```python
from build123d import *

# Parameters (mm, degrees)
F0_W     = 6
F0_H     = 21
F1_DEPTH = 4
F2_R     = 2
F3_DEPTH = 6
F4_R     = 1
F5_DEPTH = 4


with BuildPart() as f1:
    # F0 (on Top) → F1 (new body)
    with BuildSketch(Plane.XY):
        with Locations((-3, 10.5)):
            Rectangle(F0_W, F0_H)
    extrude(amount=F1_DEPTH)

    # F2 (on face) → F3 (join)
    with BuildSketch(Plane.XY.offset(4)):
        with Locations((-3, 17)):
            Circle(F2_R)
    extrude(amount=F3_DEPTH)

    # F4 (on face) → F5 (cut)
    with BuildSketch(Plane.XZ):
        with Locations((-3, 2)):
            Circle(F4_R)
    extrude(amount=-F5_DEPTH, mode=Mode.SUBTRACT)


solid = f1.part
```
The model under review builds one solid part; all positions refer to its coordinate system, in mm. A direction names the side the tool comes from. Round coordinates to 2 decimals unless told otherwise and drop trailing zeros. Write each loop counter-clockwise with the first axis right and the second up, starting at its lowest first coordinate (ties: lowest second). Pieces come first, ordered by that corner, then holes.
(1) We need section B-B on x = -3. Give the boundary of the cut face in (y, z), and give its area (3 significant figures).
(2) Wall thickness on L1, parallel to Z at x = -3, y = 1.4; L2, parallel to Z at x = -4.05, y = 10.75; L3, parallel to Y at x = -3.3, z = 2: over which ranges is each line inside the solid? List them lowest first.
(3) We need section A-A on y = 3. Give the boundary of the cut face in (x, z).
(4) Insertion check: pin 1 (1.6 mm diameter, centred on x = -3, z = 2, fed in from -Y); pin 2 (3 mm diameter, centred on x = -1, z = 3.5, fed in from -Y); pin 3 (3 mm diameter, centred on x = -4, z = 6, fed in from -Y); pin 4 (3 mm diameter, centred on x = -1.5, y = 10.5, fed in from +Z). Each pin has a flat end and moves straight along its axis. Give the tip position at first contact, or say it passes through.
(5) Mouldability with a two-part tool opening along Z and no side actions: class faces 4 (the flat face through (0, 10, 2)), 5 (the flat face through (-3, 11, 0)), 6 (the cylindrical face through (-3, 2, 1)) as +Z half, -Z half, draft (parallel to the pull), parting line (faces both ways), or undercut.
(6) We need section C-C on z = 2. Give the boundary of the cut face in (x, y).
(7) We need section D-D on y = 17. Give the boundary of the cut face in (x, z).
(8) Machinability: for faces 1 (the flat face through (-6, 10, 2)), 2 (the cylindrical face through (-3, 19, 7)), 3 (the flat face through (-3, 4, 2)), which of the approach directions +Z, -Z, +X, -X, +Y, -Y give a long, thin tool a straight path to every point of the face, cutting with its end or side? Answer none if there is none.
Findings below:
1. outline: (0, 0) - (21, 0) - (21, 4) - (19, 4) - (19, 10) - (15, 10) - (15, 4) - (0, 4) - (0, 3) - (4, 3) - (4, 1) - (0, 1) - close
1. area: 100 mm2
2. L1: z = 0 to 1, 3 to 4
2. L2: z = 0 to 4
2. L3: y = 4 to 21
3. outline: (-6, 0) - (0, 0) - (0, 4) - (-6, 4) - close; hole circle Ø2 at (-3, 2)
4. pin 1: stops at y = 4
4. pin 2: stops at y = 0
4. pin 3: stops at y = 15
4. pin 4: stops at z = 4
5. face 4: draft
5. face 5: -Z half
5. face 6: undercut
6. outline: (-6, 0) - (-4, 0) - (-4, 4) - (-2, 4) - (-2, 0) - (0, 0) - (0, 21) - (-6, 21) - close
7. outline: (-6, 0) - (0, 0) - (0, 4) - (-1, 4) - (-1, 10) - (-5, 10) - (-5, 4) - (-6, 4) - close
8. face 1: +Z, -Z, -X, +Y, -Y
8. face 2: +Z
8. face 3: -Y
